Geometry: see drawing. Coordinates: mm, zero at the bounding-box minimum. Coordinates: 2 decimals unless noted, no trailing zeros. Order: outer loops, then holes, each group sorted by start corner. A loop starts at its lowest first (then second) coordinate and runs counter-clockwise, first axis right, second up. Notation, with made-up numbers: M -35,88.25 L -8,88.25 A22 cw -8,113.25 Z; hole C -9.75,14 d11. An arc over 180 degrees is marked long. One line per item, written item: value.
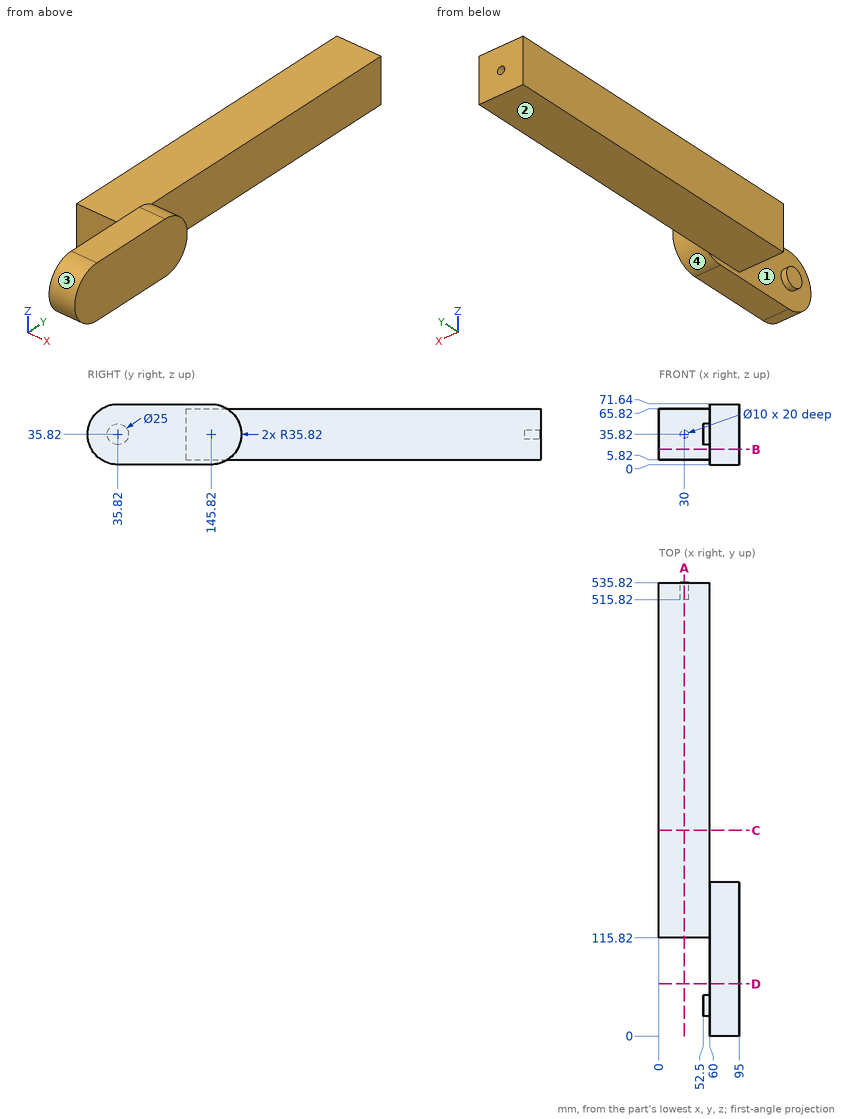
(1) Draft query along Y for the marked faces 1, 2, 3 and 4. Return one class per face: released by +Y, released by -Y, zero draft, split by the parting line, or undercut.
Data:
face 1: undercut
face 2: zero draft
face 3: released by -Y
face 4: released by +Y
(2) Ray query, line 1 (Y direction, x = 25, z = 29); line 2 (X direction, y = 236.5, z = 15); line 3 (X direction, y = 91, z = 23). Return the intervals inside material, ascending. Write a range as from..to.
Data:
line 1: y = 115.82..535.82
line 2: x = 0..60
line 3: x = 60..95
(3) Cut plane D-D on y = 61.5. Output: boundary loops of the cut face in (x, z).
Data:
outline: M 60,0 L 95,0 L 95,71.64 L 60,71.64 Z
(4) Cut plane A-A on x = 30. Output: boundary loops of the cut face in (y, z), plus the area to 3 significant figures.
Data:
outline: M 115.82,5.82 L 535.82,5.82 L 535.82,30.82 L 515.82,30.82 L 515.82,40.82 L 535.82,40.82 L 535.82,65.82 L 115.82,65.82 Z
area: 25,000 mm2
(5) Cut plane B-B on z = 18. Output: boundary loops of the cut face in (x, y).
Data:
outline: M 0,115.82 L 60,115.82 L 60,4.75 L 95,4.75 L 95,176.89 L 60,176.89 L 60,535.82 L 0,535.82 Z
(6) Cut plane C-C on y = 243. Output: boundary loops of the cut face in (x, z), plus the area to 3 significant figures.
Data:
outline: M 0,5.82 L 60,5.82 L 60,65.82 L 0,65.82 Z
area: 3,600 mm2
(7) First-contact query: pin 1 (1.5 mm diameter, centred on x = 30, y = 211.5, fed in from +Z); pin 2 (12 mm diameter, centred on x = 75, z = 14.5, fed in from -Y); pin 3 (7.5 mm diameter, centred on y = 40.5, z = 33, fed in from -X); pin 4 (1.5 mm diameter, centred on y = 225.5, z = 59.5, fed in from -X). Flat tips, straight axial feed; report the tip coordinate or a pass-through.
Data:
pin 1: stops at z = 65.82
pin 2: stops at y = 3.44
pin 3: stops at x = 52.5
pin 4: stops at x = 0
